Can you work these out from the model? Positions are in its coordinate system, mm. A direction names the side the tool comes from. Give positions to 0.01 mm unless a question says otherwise; leave off trailing zeros. Loops run counter-clockwise (first coordinate to the right, second up) from the corner with the lowest first, then second, coordinate; pieces in that order, holes last. Notation, with made-up numbers: (-8, 15.25) - (50, 15.25) arc R24 ccw to (50, 31.25) - close; hole circle Ø2 at (37, 25.25). An arc over 180 degrees is marked (long way). Write item = value, one per line.
from build123d import *

# Parameters (mm, degrees)
SKETCH_1_R          = 1.5
EXTRUDE_1_DEPTH     = 5
FILLET_1_R          = 2.5
SKETCH_3_R          = 1.5
CUT_EXTRUDE_1_DEPTH = 49


with BuildPart() as part:
    # 草图1 → 凸台-拉伸1 (new body)
    with BuildSketch(Plane.XY):
        Polygon((-14, -20), (-7, -20), (-7, -10), (-2, -10), (-2, -20), (2, -20), (2, -10), (7, -10), (7, -20), (14, -20), (14, 20), (7, 20), (7, 10), (2, 10), (2, 20), (-2, 20), (-2, 10), (-7, 10), (-7, 20), (-14, 20), align=None)
        with Locations((-11.5, 12.5)):
            Circle(SKETCH_1_R, mode=Mode.SUBTRACT)
        with Locations(Location((11.5, 12.5, 0), (0, 0, 180))):
            Circle(SKETCH_1_R, mode=Mode.SUBTRACT)
        with Locations((11.5, -12.5)):
            Circle(SKETCH_1_R, mode=Mode.SUBTRACT)
        with Locations(Location((-11.5, -12.5, 0), (0, 0, 180))):
            Circle(SKETCH_1_R, mode=Mode.SUBTRACT)
    extrude(amount=EXTRUDE_1_DEPTH)

    # 圆角1
    fillet_1_edges = [part.edges().sort_by_distance(p)[0] for p in [
        (7, -10, 2.5),
        (2, -10, 2.5),
        (-2, -10, 2.5),
        (-7, -10, 2.5),
        (7, 10, 2.5),
        (2, 10, 2.5),
        (-2, 10, 2.5),
        (-7, 10, 2.5),
    ]]
    fillet(fillet_1_edges, radius=FILLET_1_R - 0.0001)  # a hair under: the kernel refuses the full size

    # 草图3 → 切除-拉伸1 (cut)
    with BuildSketch(Plane(origin=(14, 0, 0), x_dir=(0, 0, -1), z_dir=(1, 0, 0))):
        with Locations((-2.5, 16.5)):
            Circle(SKETCH_3_R)
        with Locations(Location((-2.5, -16.5, 0), (0, 0, 90))):
            Circle(SKETCH_3_R)
    extrude(amount=-CUT_EXTRUDE_1_DEPTH, mode=Mode.SUBTRACT)


solid = part.part
Q1. Imagine slicing it at C-C, the plane y = -16.5. Write out the boundary of the cut face in (x, z), then the cut area to 3 significant figures.
Output:
outline = (-14, 0) - (-7, 0) - (-7, 1) - (-14, 1) - close; (-14, 4) - (-7, 4) - (-7, 5) - (-14, 5) - close; (-2, 0) - (2, 0) - (2, 1) - (-2, 1) - close; (-2, 4) - (2, 4) - (2, 5) - (-2, 5) - close; (7, 0) - (14, 0) - (14, 1) - (7, 1) - close; (7, 4) - (14, 4) - (14, 5) - (7, 5) - close
area = 36.0 mm2
Q2. We'd pull the mould along Y, two halves only. Please class faces 1 (the flat face through (7, 15, 1)), 2 (the cylindrical face through (2.713, -10.752, 2.535)), 3 (the cylindrical face through (10, -12.43, 2.46)): released by +Y, released by -Y, zero draft, split by the parting line, or undercut.
Output:
face_1 = zero draft
face_2 = released by -Y
face_3 = undercut
Q3. Imagine slicing it at B-B, the plane z = 4.4. Give the number of separate pieces and of enclosed holes in the cut face, then the cut area to 3 significant figures.
Output:
separate_pieces = 1
enclosed_holes = 4
area = 902 mm2
Q4. Imagine slicing it at D-D, the plane x = 7.5. Write out the boundary of the cut face in (y, z), then the cut area to 3 significant figures.
Output:
outline = (-20, 0) - (20, 0) - (20, 5) - (-20, 5) - close; hole circle Ø3 at (-16.5, 2.5); hole circle Ø3 at (16.5, 2.5)
area = 186 mm2
Q5. For pin 1 (2.5 mm diameter, centred on y = -16.5, z = 2.5, fed in from -X), with a flat end and sliding along its axis, tell me the tip position at first contact or that it passes through.
Output:
pin_1 = through
Q6. Which directions (+Z, -Z, +X, -X, +Y, -Y) give clear straight access to the entire face, cutting with the end or side of a thin tool? Please do faces 4 (the cylindrical face through (10.549, 17.987, 2.695)), 5 (the flat face through (7, -15, 1)), 6 (the cylindrical face through (-6.287, 10.752, 2.535)).
Output:
face_4 = +X, -X
face_5 = +Z, -Z, -Y
face_6 = +Z, -Z, +Y
Q7. Imagine slicing it at A-A, the plane x = -11.5. Write out the boundary of the cut face in (y, z).
Output:
outline = (-20, 0) - (-14, 0) - (-14, 5) - (-20, 5) - close; (-11, 0) - (11, 0) - (11, 5) - (-11, 5) - close; (14, 0) - (20, 0) - (20, 5) - (14, 5) - close; hole circle Ø3 at (-16.5, 2.5); hole circle Ø3 at (16.5, 2.5)
Q8. I need wall thicknesses on L1, parallel to X at y = -15, z = 3.8; L2, parallel to Y at x = 11.5, z = 2.85; L3, parallel to X at y = -13, z = 1.4. Which ranges of each line are inside material? Lowest first, please.
Output:
L1 = -14 to -7, -2 to 2, 7 to 14
L2 = -20 to -17.96, -15.04 to -14, -11 to 11, 14 to 15.04, 17.96 to 20
L3 = -14 to -12.91, -10.09 to -7, -2 to 2, 7 to 10.09, 12.91 to 14
